Part model, mm, in its own coordinate system. A direction names the side the tool comes from. Give positions to 0.01 mm unless a question says otherwise; leave off trailing zeros. Order: outer loops, then holes, each group sorted by start corner. A loop starts at its lowest first (then second) coordinate and runs counter-clockwise, first axis right, second up. Notation, with made-up numbers: M -39.75,-26 L 14.25,-26 A32 cw 14.25,13 Z; hole C 72.5,6 d7. An arc over 180 degrees is marked long. Write each question's results on one line, items separated by ' | '. Start each with the question number.
Solid Edge part; units mm, degrees
sketch "Sketch1" plane through (0, 0, 0) normal (0, 0, 1) x (1, 0, 0)
  circle A0 centre (0, 0) radius 15
extrude "Protrusion1" add sketch "Sketch1" along normal blind 5
fillet "Round_1" [suppressed]
sketch "Sketch2" plane through (0, 0, 0) normal (0, 0, -1) x (-1, 0, 0)
  circle A0 centre (5.3033, 5.3033) radius 2
extrude "Protrusion2" add sketch "Sketch2" along normal blind 20
pattern_circular "Pattern1" count 4 over 360 about axis through (0, 0, 0) along (0, 0, 1) of "Protrusion2"
fillet "Round1" [suppressed]
extrude "Protrusion3" [suppressed]
extrude "Protrusion4" [suppressed]
fillet "Round_5" [suppressed]
fillet "Round_6" [suppressed]
extrude "ExtrudedProtrusion_9" [suppressed]
extrude "ExtrudedCutout_2" [suppressed]
fillet "Round_7" [suppressed]
fillet "Round_8" [suppressed]
extrude "ExtrudedProtrusion_10" [suppressed]
(1) Saw through at C-C on z = 2.5. Give the cut face in (x, y), plus the area to 3 significant figures.
(2) Pull direction Y, two halves, no side cores. Call faces 3 (the flat face through (0, 0, 5)), 4 (the cylindrical face through (-14.985, -0.66, 2.465)), 5 (the cylindrical face through (6.5, 3.7, -9.9)): +Y half, -Y half, draft (parallel to the pull), parting line (faces both ways), or undercut.
(3) Drop flat-ended pins along their axis: P1, Ø6, axis at x = 5.5, z = -17, coming from the +Y side; P2, Ø4, axis at x = -10.5, y = 0, coming from the -Z side; P3, Ø8, axis at y = 1, z = -12.5, coming from the +X side. Give the stop position or say it passes through.
(4) Saw through at B-B on y = 4.75. Give the cut face in (x, z).
(5) Saw through at D-D on z = -10.25. Give the cut face in (x, y).
(6) Tool access for faces 1 (the flat face through (5, 5, -20)), 2 (the flat face through (0, 0, 0)): list every direction of +Z, -Z, +X, -X, +Y, -Y with a clear straight run to the whole face (end or side of a thin tool).
(7) Saw through at A-A on x = 0. Give the cut face in (y, z), plus the area to 3 significant figures.
(8) Probe L1, parallel to Y at x = -5.25, z = -10.5; L2, parallel to X at y = -5.5, z = -18.5; L3, parallel to Z at x = 0, y = 10.5. List the from-to ranges inside material, lowest first.
Taken from the geometry:
1) outline: C 0,0 d30 | area: 707 mm²
2) face 3: draft | face 4: parting line | face 5: undercut
3) P1: stops at y = 7.3 | P2: stops at z = 0 | P3: stops at x = 7.28
4) outline: M -14.23,0 L -7.23,0 L -7.23,-20 L -3.38,-20 L -3.38,0 L 3.38,0 L 3.38,-20 L 7.23,-20 L 7.23,0 L 14.23,0 L 14.23,5 L -14.23,5 Z
5) outline: C -5.3,-5.3 d4; C -5.3,5.3 d4; C 5.3,-5.3 d4; C 5.3,5.3 d4
6) face 1: -Z, +X, -X, +Y, -Y | face 2: -Z
7) outline: M -15,0 L 15,0 L 15,5 L -15,5 Z | area: 150 mm²
8) L1: y = -7.3 to -3.3, 3.3 to 7.3 | L2: x = -7.29 to -3.31, 3.31 to 7.29 | L3: z = 0 to 5
